Verification items for the finished model (mm, model axes). Face numbers are marked on the shaded views. A direction names the side the tool comes from. Give positions to 0.01 mm unless a question says otherwise; leave off trailing zeros. Order: outer loops, then holes, each group sorted by start corner. A loop starts at its lowest first (then second) coordinate and runs counter-clockwise, first axis right, second up.
(1) Sectioned sample at A-A on z = -40.5. Record the cut outline in (x, y) (1 decimal).
(2) Sectioned sample at C-C on x = -110. Record the cut outline in (y, z), plus the area to 3 significant figures.
(3) Sectioned sample at D-D on x = -74.5. Record the cut outline in (y, z).
(4) Scan lines: L1, parallel to X at y = 0.5, z = -23.5 (3 decimals); L2, parallel to Z at x = 32, y = 4.75; L3, parallel to Y at x = -126.5, z = -29.5. Record each from-to range of solid material in increasing order.
(5) Gauge pin test, flat ends, axial feed: pin 1 (1 mm diameter, centred on y = 7.5, z = -12.5, fed in from -X); pin 2 (24 mm diameter, centred on x = -109, z = -34.5, fed in from -Y); pin 3 (10 mm diameter, centred on y = 12.5, z = -17.5, fed in from -X). Record the tip position at first contact, or that the pin passes through.
(6) Mould release check, pull along X, two halves, no side actions. Record for the marked faces 6, 7 and 8: pulls with the +X half, pulls with the -X half, needs draft (parallel to the pull), parting line crosses it, or undercut.
(7) Access from +Z, -Z, +X, -X, +Y, -Y to the whole of each face (thin tool, end or side, straight path). Record for the marked faces 1, 2, 3, 4 and 5.
(8) Sectioned sample at B-B on y = -13.5. Record the cut outline in (x, z).
```python
from build123d import *

# Parameters (mm, degrees)
BOSS_EXTRUDE1_DEPTH   = 44
BOSS_EXTRUDE2_START   = -10
BOSS_EXTRUDE2_DEPTH   = 24
BOSS_EXTRUDE3_START   = -22
BOSS_EXTRUDE3_DEPTH   = 22
BOSS_EXTRUDE4_START   = -29
BOSS_EXTRUDE4_DEPTH   = 15
FILLET1_RADIUS        = 12
FILLET1_LENGTH        = 9
FILLET2_RADIUS        = 12
FILLET2_LENGTH        = 9
F_6_0MM_DOWEL_HOLE1_D = 6


with BuildPart() as part:
    # Sketch1 → Boss-Extrude1 (new body)
    with BuildSketch(Plane.XY):
        with BuildLine():
            Line((15.835957699, 1), (24.979991994, 1))
            ThreePointArc((24.979991994, 1), (-25, 0), (24.979991994, -1))
            Line((24.979991994, -1), (15.835957699, -1))
            ThreePointArc((15.835957699, -1), (-15.8675, 0), (15.835957699, 1))
        make_face()
    extrude(amount=-BOSS_EXTRUDE1_DEPTH)

    # Sketch1<3> → Boss-Extrude2 (add)
    with BuildSketch(Plane.XY.offset(BOSS_EXTRUDE2_START)):
        with BuildLine():
            Line((44, 10), (22.912878475, 10))
            ThreePointArc((22.912878475, 10), (24.365585575, 5.596270148), (24.979991994, 1))
            Line((24.979991994, 1), (44, 1))
            Line((44, 1), (44, 10))
        make_face()
        with BuildLine():
            ThreePointArc((24.979991994, -1), (24.365585575, -5.596270148), (22.912878475, -10))
            Line((22.912878475, -10), (44, -10))
            Line((44, -10), (44, -1))
            Line((44, -1), (24.979991994, -1))
        make_face()
    extrude(amount=-BOSS_EXTRUDE2_DEPTH)



with BuildPart() as body_2:
    # Sketch1<4> → Boss-Extrude3 (new body)
    with BuildSketch(Plane.XY.offset(BOSS_EXTRUDE3_START)):
        with BuildLine():
            Line((-140, 20), (-90, 20))
            ThreePointArc((-90, 20), (-70, 0), (-90, -20))
            Line((-90, -20), (-140, -20))
            ThreePointArc((-140, -20), (-160, 0), (-140, 20))
        make_face()
        with BuildLine():
            Line((-140, 6), (-90, 6))
            ThreePointArc((-90, 6), (-84, 0), (-90, -6))
            Line((-90, -6), (-140, -6))
            ThreePointArc((-140, -6), (-146, 0), (-140, 6))
        make_face(mode=Mode.SUBTRACT)
    extrude(amount=-BOSS_EXTRUDE3_DEPTH)


with BuildPart() as part_1:
    add(part.part)

    add(body_2.part)  # Boss-Extrude4 merges body 2
    # Sketch1<5> → Boss-Extrude4 (add)
    with BuildSketch(Plane.XY.offset(BOSS_EXTRUDE4_START)):
        with BuildLine():
            Line((-1.388888889, 24.961389938), (-90.555984888, 20))
            Line((-90.555984888, 20), (-90, 20))
            ThreePointArc((-90, 20), (-70, 0), (-90, -20))
            Line((-90, -20), (-90.555984888, -20))
            Line((-90.555984888, -20), (-1.388888889, -24.961389938))
            ThreePointArc((-1.388888889, -24.961389938), (-25, 0), (-1.388888889, 24.961389938))
        make_face()
    extrude(amount=-BOSS_EXTRUDE4_DEPTH)

    # Fillet1: full round fillet: the end face becomes a half cylinder, R = half its width
    fillet1_face = Plane((44, 5.5, -22), x_dir=(0, 1, 0), z_dir=(1, 0, 0))  # on the end face: x along it, z out of the body
    fillet1_slab = fillet1_face.offset(-FILLET1_RADIUS / 2) * Box(FILLET1_LENGTH, 2 * FILLET1_RADIUS, FILLET1_RADIUS, mode=Mode.PRIVATE)  # the body's end, R deep
    fillet1_round = Plane((32, 5.5, -22), x_dir=(1, 0, 0), z_dir=(0, 1, 0)) * Cylinder(FILLET1_RADIUS, FILLET1_LENGTH, mode=Mode.PRIVATE)  # its axis R under the face
    add(fillet1_slab - fillet1_round, mode=Mode.SUBTRACT)

    # Fillet2: full round fillet: the end face becomes a half cylinder, R = half its width
    fillet2_face = Plane((44, -5.5, -22), x_dir=(0, -1, 0), z_dir=(1, 0, 0))  # on the end face: x along it, z out of the body
    fillet2_slab = fillet2_face.offset(-FILLET2_RADIUS / 2) * Box(FILLET2_LENGTH, 2 * FILLET2_RADIUS, FILLET2_RADIUS, mode=Mode.PRIVATE)  # the body's end, R deep
    fillet2_round = Plane((32, -5.5, -22), x_dir=(1, 0, 0), z_dir=(0, -1, 0)) * Cylinder(FILLET2_RADIUS, FILLET2_LENGTH, mode=Mode.PRIVATE)  # its axis R under the face
    add(fillet2_slab - fillet2_round, mode=Mode.SUBTRACT)

    # Ø6.0mm Dowel Hole1 (through all)
    with Locations(Plane(origin=(32, 10, -22), x_dir=(1, 0, 0), z_dir=(0, 1, 0))):
        with Locations((0, 0)):
            Hole(F_6_0MM_DOWEL_HOLE1_D / 2)


solid = part_1.part
```
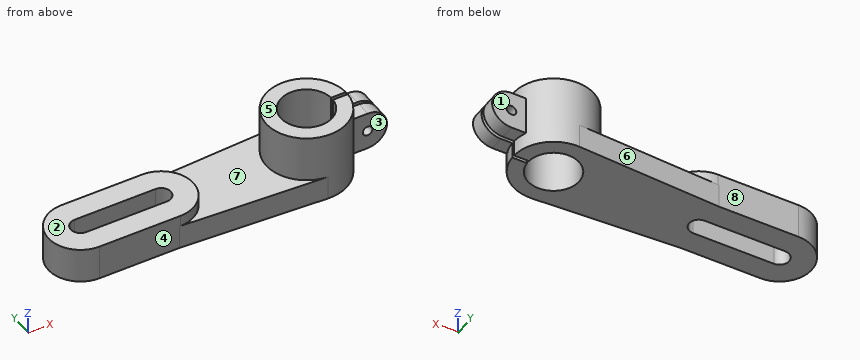
Ans:
1. outline: (-140, -20) - (-90.6, -20) - (-1.4, -25) arc R25 ccw to (25, -1) - (15.8, -1) arc R15.9 cw (long way) to (15.8, 1) - (25, 1) arc R25 ccw to (-1.4, 25) - (-90.6, 20) - (-140, 20) arc R20 ccw to start; hole (-140, -6) - (-90, -6) arc R6 ccw to (-90, 6) - (-140, 6) arc R6 ccw to start
2. outline: (-20, -44) - (-6, -44) - (-6, -22) - (-20, -22) - close; (6, -44) - (20, -44) - (20, -22) - (6, -22) - close
2. area: 616 mm2
3. outline: (-20.89, -44) - (20.89, -44) - (20.89, -29) - (12.64, -29) - (12.64, -22) - (-12.64, -22) - (-12.64, -29) - (-20.89, -29) - close
4. L1: x = -159.994 to -145.979, -84.021 to -70.006, -24.995 to -15.86
4. L2: z = -34 to -25, -19 to -10
4. L3: y = -20 to -6, 6 to 20
5. pin 1: stops at x = -24
5. pin 2: stops at y = -20
5. pin 3: stops at x = -157.13
6. face 6: pulls with the -X half
6. face 7: undercut
6. face 8: needs draft
7. face 1: +Z, -Z, +X, +Y
7. face 2: +Z, -X, +Y, -Y
7. face 3: +Z, -Z, +X, -Y
7. face 4: +Z, -Z, -X, -Y
7. face 5: +Z, +X, -X, +Y, -Y
8. outline: (-154.76, -44) - (-8.34, -44) - (-8.34, 0) - (-21.04, 0) - (-21.04, -29) - (-75.24, -29) - (-75.24, -22) - (-154.76, -22) - close; (8.34, -44) - (21.04, -44) - (21.04, 0) - (8.34, 0) - close
